from build123d import *

# Parameters (mm, degrees)
SKETCH1_R           = 9
BOSS_EXTRUDE1_DEPTH = 3
CUT_EXTRUDE1_DEPTH  = 14.076696831
CIRPATTERN1_COUNT   = 10
CUT_EXTRUDE3_DEPTH  = 13.851135167


with BuildPart() as part:
    # Sketch1 → Boss-Extrude1 (new body)
    with BuildSketch(Plane.XY):
        Circle(SKETCH1_R)
    extrude(amount=BOSS_EXTRUDE1_DEPTH)

    # Sketch2 → Cut-Extrude1 (cut, through all)
    with BuildSketch(Plane.XY.offset(3)):
        with BuildLine():
            ThreePointArc((-2.41833102, 8.669006579), (0, 9), (2.41833102, 8.669006579))
            ThreePointArc((2.41833102, 8.669006579), (1.091553585, 7.387918037), (0.76495134, 5.572743889))
            ThreePointArc((0.76495134, 5.572743889), (0, 5.625), (-0.76495134, 5.572743889))
            ThreePointArc((-0.76495134, 5.572743889), (-1.091553585, 7.387918037), (-2.41833102, 8.669006579))
        make_face()
    cut_extrude1 = extrude(amount=-CUT_EXTRUDE1_DEPTH, mode=Mode.SUBTRACT)

    # CirPattern1: Cut-Extrude1 ×10 about axis
    cirpattern1_axis = Axis((0, 0, 0), (0, 0, 1))
    for i in range(1, CIRPATTERN1_COUNT):
        add(cut_extrude1.rotate(cirpattern1_axis, i * 360 / CIRPATTERN1_COUNT), mode=Mode.SUBTRACT)

    # Sketch4 → Cut-Extrude3 (cut, through all)
    with BuildSketch(Plane.XY.offset(3)):
        with BuildLine():
            Line((-1.322875656, 1.5), (1.322875656, 1.5))
            ThreePointArc((1.322875656, 1.5), (0, -2), (-1.322875656, 1.5))
        make_face()
    extrude(amount=-CUT_EXTRUDE3_DEPTH, mode=Mode.SUBTRACT)


solid = part.part
Could you check a few things on this model? Use its own coordinates, in mm. Give positions to 0.01 mm unless a question says otherwise; leave off trailing zeros. Loops run counter-clockwise (first coordinate to the right, second up) from the corner with the lowest first, then second, coordinate; pieces in that order, holes last. Notation, with made-up numbers: (63, -37) -> (97, -37) arc R19 ccw to (97, -4) -> close; hole circle Ø2 at (6.25, 7.25). An arc over 180 degrees is marked (long way). Answer as CSV lines item,"result". Start each with the question number.
(1) I'm going to push flat-ended pins straight in: pin 1 Ø1.3 at (x, z) = (0, 2) entering from -Y (3 decimals); pin 2 Ø1.5 at (y, z) = (3.5, 1) entering from +X. Where does each tip first touch, or does it pass through?
(2) If we section it at C-C on y = 4.5: Write out the boundary of the cut face in (x, z) (3 decimals), then the cut area to 3 significant figures.
(3) If we section it at D-D on x = -6.75: Write out the boundary of the cut face in (y, z), then the cut area to 3 significant figures.
(4) We'd pull the mould along X, two halves only. Please class faces 1 (the cylindrical face through (3.463, -6.645, 1.521)), 2 (the cylindrical face through (0, -2, 2)), 3 (the flat face through (0, 2, 0)): released by +X, released by -X, zero draft, split by the parting line, or undercut.
(5) I need wall thicknesses on probe 1 along Y at (x, z) = (0, 1.7) (3 decimals); probe 2 along X at (y, z) = (0, 1.6); probe 3 along Y at (x, z) = (-3.25, 1.15). Which ranges of each line are inside material? Lowest first, please.
(6) If we section it at A-A on y = 0: Write out the boundary of the cut face in (x, z).
(7) If we section it at B-B on x = 0: Write out the boundary of the cut face in (y, z) (3 decimals), then the cut area to 4 significant figures.
Computed:
1,pin 1,"stops at y = -5.625"
1,pin 2,"stops at x = 7.3"
2,outline,"(-7.389, 0) -> (-4.185, 0) -> (-4.185, 3) -> (-7.389, 3) -> close; (-3.375, 0) -> (3.375, 0) -> (3.375, 3) -> (-3.375, 3) -> close; (4.185, 0) -> (7.389, 0) -> (7.389, 3) -> (4.185, 3) -> close"
2,area,"39.5 mm2"
3,outline,"(-5.63, 0) -> (-3.39, 0) -> (-3.39, 3) -> (-5.63, 3) -> close; (-1.29, 0) -> (1.29, 0) -> (1.29, 3) -> (-1.29, 3) -> close; (3.39, 0) -> (5.63, 0) -> (5.63, 3) -> (3.39, 3) -> close"
3,area,"21.2 mm2"
4,face 1,"undercut"
4,face 2,"undercut"
4,face 3,"zero draft"
5,probe 1,"y = -5.625 to -2, 1.5 to 5.625"
5,probe 2,"x = -9 to -2, 2 to 9"
5,probe 3,"y = -8.2 to -5.86, -4.59 to 4.59, 5.86 to 8.2"
6,outline,"(-9, 0) -> (-2, 0) -> (-2, 3) -> (-9, 3) -> close; (2, 0) -> (9, 0) -> (9, 3) -> (2, 3) -> close"
7,outline,"(-5.625, 0) -> (-2, 0) -> (-2, 3) -> (-5.625, 3) -> close; (1.5, 0) -> (5.625, 0) -> (5.625, 3) -> (1.5, 3) -> close"
7,area,"23.25 mm2"
